CAD build for the part. Positions are in the model's coordinates, mm. A direction names the side the tool comes from. Give positions to 0.01 mm unless a question says otherwise; leave off trailing zeros. Order: outer loops, then holes, each group sorted by start corner. A loop starts at its lowest first (then second) coordinate and runs counter-clockwise, first axis right, second up. Notation, with made-up numbers: M 85,-36 L 110,-36 A32 ccw 110,-4 Z; hole C 13.5,36.5 d1. An arc over 180 degrees is marked long. Put each result on its own line as item: value. Start each with the question number.
1) Drill centre lines: line 1 (Y direction, x = 0, z = 2); line 2 (Y direction, x = 0.25, z = 8.5); line 3 (Y direction, x = 0.5, z = 6.75). Where is each one in solid material? Low to high. Write a range as [from, to].
2) Pin check, flat tips, straight feed: pin 1 (4.5 mm diameter, centred on x = 0, y = 0, fed in from +Z); pin 2 (3 mm diameter, centred on x = 0.5, y = -1, fed in from -Z); pin 3 (1.5 mm diameter, centred on x = -1.5, z = 5.5, fed in from +Y). Stop position of each tip, or through.
3) Tool access for faces 5 (the face through (-2, -16, 7)), 6 (the face through (-2.39, 1.4, 1.48)), 7 (the face through (0, 19, 5)): list every direction of +Z, -Z, +X, -X, +Y, -Y with a clear straight run to the whole face (end or side of a thin tool).
4) Cut at B-B (z = 4.5). Write the cut outline in (x, y).
5) Two-plate mould, pull along X, no slides. Class faces 1 (the face through (0, -2, 5)), 2 (the face through (1, -18, 10)), 3 (the face through (-3.89, -15.93, 1.48)), 4 (the face through (-2.406, -1.375, 1.479)): released by +X, released by -X, zero draft, split by the parting line, or undercut.
6) Cut at A-A (z = 8.5). Write the cut outline in (x, y), and give its area (3 significant figures).
7) Cut at C-C (z = 2). Write the cut outline in (x, y).
8) Cut at D-D (y = -15.5). Write the cut outline in (x, z), and give its area (3 significant figures).
Autodesk Inventor part; units mm, degrees
ref_plane "YZ Plane" through (0, 0, 0) normal (1, 0, 0) x (0, 1, 0)
ref_plane "XZ Plane" through (0, 0, 0) normal (0, 1, 0) x (-1, 0, 0)
ref_plane "XY Plane" through (0, 0, 0) normal (0, 0, 1) x (1, 0, 0)
sketch "Sketch1" plane through (0, 0, 0) normal (0, 0, 1) x (1, 0, 0)
  line L0 (0, -15) -> (0, 15) construction
  line L1 (-4, -15) -> (-4, 15)
  line L2 (4, 15) -> (4, -15)
  arc A0 (-4, -15) -> (0, -19) centre (0, -15) ccw
  arc A1 (4, 15) -> (-4, 15) centre (0, 15) ccw
  line L3 (4, -15) -> (0, -15)
  line L4 (-4, -11) -> (-4, -19)
  line L5 (-4, -19) -> (4, -19)
  line L6 (4, -19) -> (4, -15)
  point P0 (0, 0)
  point P1 (0, 0)
  dimension "d0" = 4
  dimension "d17" = 30
extrude "Extrusion1" add sketch "Sketch1" along normal blind 10 contours L1 A1 L2 L6 L5 A0
sketch "Sketch2" plane through (0, 0, 10) normal (0, 0, 1) x (1, 0, 0)
  line L0 (-4, 15) -> (-4, -15)
  arc A0 (-4, -15) -> (0, -19) centre (0, -15) ccw
  line L1 (4, -19) -> (4, 15)
  arc A1 (4, 15) -> (-4, 15) centre (0, 15) ccw
  circle A2 centre (0, 0) radius 13
  circle A3 centre (0, 0) radius 3.75
  line L2 (0, -19) -> (4, -19)
  dimension "d3" = 26
  dimension "d4" = 7.5
extrude "Extrusion2" cut sketch "Sketch2" against normal blind 7 contours A2 L1 L0 | L0 A2 | A2 L1
sketch "Sketch3" plane through (0, 0, 10) normal (0, 0, 1) x (1, 0, 0)
  circle A0 centre (0, 0) radius 3.75
  circle A1 centre (0, 0) radius 2
  line L0 (-4, -12.3693) -> (-4, -15)
  line L1 (4, 12.3693) -> (4, 15)
  arc A2 (4, 12.3693) -> (-4, 12.3693) centre (0, 0) ccw
  arc A3 (4, 15) -> (-4, 15) centre (0, 15) ccw
  arc A4 (-4, -12.3693) -> (4, -12.3693) centre (0, 0) ccw
  arc A5 (-4, -15) -> (0, -19) centre (0, -15) ccw
  line L2 (0, -19) -> (4, -19)
  line L3 (-4, 15) -> (-4, 12.3693)
  line L4 (4, -19) -> (4, -12.3693)
  dimension "d7" = 4
extrude "Extrusion3" cut sketch "Sketch3" against normal through all contours A1
sketch "Sketch4" plane through (0, 0, 0) normal (0, 0, -1) x (-1, 0, 0)
  circle A0 centre (0, 0) radius 2
  line L0 (4, -15) -> (4, 15)
  arc A1 (4, 15) -> (-4, 15) centre (0, 15) ccw
  line L1 (-4, 15) -> (-4, -19)
  arc A2 (0, -19) -> (4, -15) centre (0, -15) ccw
  circle A3 centre (0, 0) radius 2
  line L2 (1.5898, -2.7772) -> (-1.6102, -2.7654)
  line L3 (-1.6102, -2.7654) -> (-3.2, 0.0118)
  line L4 (-3.2, 0.0118) -> (-1.5898, 2.7772)
  line L5 (-1.5898, 2.7772) -> (1.6102, 2.7654)
  line L6 (1.6102, 2.7654) -> (3.2, -0.0118)
  line L7 (3.2, -0.0118) -> (1.5898, -2.7772)
  circle A4 centre (0, 0) radius 3.2
  line L8 (-4, -19) -> (0, -19)
  dimension "d10" = 6.4
extrude "Extrusion4" cut sketch "Sketch4" against normal blind 3 contours L2 L3 L4 L5 L6 L7
sketch "Sketch8" plane through (0, 0, 10) normal (0, 0, 1) x (1, 0, 0)
  arc A0 (4, 12.3693) -> (-4, 12.3693) centre (0, 0) ccw
  line L0 (4, 12.3693) -> (4, 15)
  arc A1 (4, 15) -> (-4, 15) centre (0, 15) ccw
  line L1 (-4, 15) -> (-4, 12.3693)
  circle A2 centre (0, 16) radius 1.75
  dimension "d28" = 3.5
  dimension "d40" = 1
  dimension "d41" = 5.402
extrude "Extrusion8" cut sketch "Sketch8" against normal through all contours A2
sketch "Sketch10" plane through (0, 0, 10) normal (0, 0, 1) x (1, 0, 0)
  circle A0 centre (0, 0) radius 2
  circle A1 centre (0, 0) radius 2
  circle A2 centre (0, 0) radius 3.75
extrude "Extrusion10" cut sketch "Sketch10" against normal blind 3
sketch "Sketch12" plane through (0, 0, 10) normal (0, 0, 1) x (1, 0, 0)
  arc A0 (-4, -12.3693) -> (4, -12.3693) centre (0, 0) ccw
  line L0 (-4, -12.3693) -> (-4, -15)
  arc A1 (-4, -15) -> (0, -19) centre (0, -15) ccw
  line L1 (0, -19) -> (4, -19)
  line L2 (4, -19) -> (4, -12.3693)
  line L3 (4, -19) -> (4, -24)
  line L4 (4, -24) -> (0, -24)
  line L5 (0, -24) -> (-3.5832, -16.7778)
  arc A2 (-4, -15) -> (0, -19) centre (0, -15) ccw
  arc A3 (-4, -15) -> (0, -19) centre (0, -15) ccw
  line L6 (0, -19) -> (4, -19)
  dimension "d42" = 5
extrude "Extrusion11" add sketch "Sketch12" against normal up to surface (10 mm away) from surface at 0 contours L3 L4 L5 A1 L1
sketch "Sketch9" plane through (-4, -15, 0) normal (-1, 0, 0) x (0, 0, 1)
  line L0 (0, 0) -> (10, 0)
  line L1 (5, 0) -> (5, -2.3027) construction
  line L2 (3, 0) -> (3, -2.3027)
  line L3 (7, -2.3027) -> (7, 0)
  arc A0 (7, 0) -> (3, 0) centre (5, 0) ccw
  arc A1 (3, -2.3027) -> (7, -2.3027) centre (5, -2.3027) ccw
  line L4 (3, 2.6307) -> (3, 27.3693)
  point P0 (0, 15)
  point P1 (5, -1.1513)
  dimension "d31" = 4
  dimension "d34" = 2
  dimension "d45" = 1.1514
extrude "Extrusion9" cut sketch "Sketch9" against normal blind 4
fillet "Fillet4" radius 2 2 edges at (0, -24, 5) (4, -24, 5)
properties part number "rodamiento0.3"
Solution:
1. line 1: [-23.57, -2.77], [2.77, 14.25], [17.75, 19]
1. line 2: [-23.74, -13], [13, 14.27], [17.73, 18.99]
1. line 3: [-23.86, -12.99], [-3.72, -1.94], [1.94, 3.72], [12.99, 14.32], [17.68, 18.97]
2. pin 1: z = 7
2. pin 2: z = 3
2. pin 3: y = 18.93
3. face 5: -X
3. face 6: -Z
3. face 7: +Z, -Z, +Y
4. outline: M -4,-13.06 L 0,-13.06 L 0,-19.24 L -2.36,-19.24 L -0.55,-22.89 A2 ccw 1.24,-24 L 2,-24 A2 ccw 4,-22 L 4,-12.37 A13 cw -4,-12.37 Z; M -4,12.37 A13 cw 4,12.37 L 4,15 A4 ccw -4,15 Z; C 0,0 d7.5; hole C 0,0 d4; hole C 0,16 d3.5
5. face 1: undercut
5. face 2: zero draft
5. face 3: released by -X
5. face 4: undercut
6. outline: M -4,-15 A4 ccw -3.58,-16.78 L -0.55,-22.89 A2 ccw 1.24,-24 L 2,-24 A2 ccw 4,-22 L 4,-12.37 A13 cw -4,-12.37 Z; M -4,12.37 A13 cw 4,12.37 L 4,15 A4 ccw -4,15 Z; hole C 0,16 d3.5
6. area: 106 mm²
7. outline: M -4,-15 A4 ccw -3.58,-16.78 L -0.55,-22.89 A2 ccw 1.24,-24 L 2,-24 A2 ccw 4,-22 L 4,15 A4 ccw -4,15 Z; hole M -3.2,-0.01 L -1.59,-2.78 L 1.61,-2.77 L 3.2,0.01 L 1.59,2.78 L -1.61,2.77 Z; hole C 0,16 d3.5
8. outline: M -3.97,0 L 4,0 L 4,10 L -3.97,10 L -3.97,7 L 0,7 L 0,3 L -3.97,3 Z
8. area: 63.8 mm²
